```python
from build123d import *

# Parameters (mm, degrees)
F1_DEPTH = 2
F2_R     = 1
F3_DEPTH = 2.001


with BuildPart() as f1:
    # F0 (on Top) → F1 (new body)
    with BuildSketch(Plane.XY):
        with BuildLine():
            ThreePointArc((9.772306, -2.121802), (9.942913, -1.066992), (10, 0))
            ThreePointArc((10, 0), (9.999976, 0.02183), (9.999905, 0.043659))
            ThreePointArc((9.999905, 0.043659), (9.945219, 1.045285), (9.79046, 2.036392))
            ThreePointArc((9.79046, 2.036392), (9.510565, 3.09017), (9.11761, 4.107212))
            ThreePointArc((9.11761, 4.107212), (8.660254, 5), (8.115755, 5.842476))
            ThreePointArc((8.115755, 5.842476), (7.431448, 6.691306), (6.658797, 7.460591))
            ThreePointArc((6.658797, 7.460591), (5.877853, 8.09017), (5.037762, 8.638342))
            ThreePointArc((5.037762, 8.638342), (4.067366, 9.135455), (3.048618, 9.523966))
            ThreePointArc((3.048618, 9.523966), (2.079117, 9.781476), (1.088694, 9.940561))
            ThreePointArc((1.088694, 9.940561), (0, 10), (-1.088694, 9.940561))
            ThreePointArc((-1.088694, 9.940561), (-2.079117, 9.781476), (-3.048618, 9.523966))
            ThreePointArc((-3.048618, 9.523966), (-4.067366, 9.135455), (-5.037762, 8.638342))
            ThreePointArc((-5.037762, 8.638342), (-5.877853, 8.09017), (-6.658797, 7.460591))
            ThreePointArc((-6.658797, 7.460591), (-7.431448, 6.691306), (-8.115755, 5.842476))
            ThreePointArc((-8.115755, 5.842476), (-8.660254, 5), (-9.11761, 4.107212))
            ThreePointArc((-9.11761, 4.107212), (-9.510565, 3.09017), (-9.79046, 2.036392))
            ThreePointArc((-9.79046, 2.036392), (-9.945219, 1.045285), (-9.999905, 0.043659))
            ThreePointArc((-9.999905, 0.043659), (-9.945219, -1.045285), (-9.772306, -2.121802))
            ThreePointArc((-9.772306, -2.121802), (-9.510565, -3.09017), (-9.153125, -4.027443))
            ThreePointArc((-9.153125, -4.027443), (-8.660254, -5), (-8.064431, -5.913117))
            ThreePointArc((-8.064431, -5.913117), (-7.431448, -6.691306), (-6.723687, -7.402164))
            ThreePointArc((-6.723687, -7.402164), (-5.877853, -8.09017), (-4.962143, -8.682001))
            ThreePointArc((-4.962143, -8.682001), (-4.067366, -9.135455), (-3.131663, -9.496983))
            ThreePointArc((-3.131663, -9.496983), (-2.079117, -9.781476), (-1.001855, -9.949688))
            ThreePointArc((-1.001855, -9.949688), (0, -10), (1.001855, -9.949688))
            ThreePointArc((1.001855, -9.949688), (2.079117, -9.781476), (3.131663, -9.496983))
            ThreePointArc((3.131663, -9.496983), (4.067366, -9.135455), (4.962143, -8.682001))
            ThreePointArc((4.962143, -8.682001), (5.877853, -8.09017), (6.723687, -7.402164))
            ThreePointArc((6.723687, -7.402164), (7.431448, -6.691306), (8.064431, -5.913117))
            ThreePointArc((8.064431, -5.913117), (8.660254, -5), (9.153125, -4.027443))
            ThreePointArc((9.153125, -4.027443), (9.510565, -3.09017), (9.772306, -2.121802))
        make_face()
        with BuildLine():
            ThreePointArc((9.999905, 0.043659), (9.999976, 0.02183), (10, 0))
            ThreePointArc((10, 0), (9.942913, -1.066992), (9.772306, -2.121802))
            ThreePointArc((9.772306, -2.121802), (10.85461, -2.093182), (11.881999, -1.751603))
            Line((11.881999, -1.751603), (11.934263, -1.254342))
            Line((11.934263, -1.254342), (11.986527, -0.757081))
            ThreePointArc((11.986527, -0.757081), (11.052608, -0.209359), (9.999905, 0.043659))
        make_face()
        with BuildLine():
            ThreePointArc((9.11761, 4.107212), (9.510565, 3.09017), (9.79046, 2.036392))
            ThreePointArc((9.79046, 2.036392), (10.767554, 2.502751), (11.567187, 3.232676))
            Line((11.567187, 3.232676), (11.412678, 3.708204))
            Line((11.412678, 3.708204), (11.25817, 4.183732))
            ThreePointArc((11.25817, 4.183732), (10.182214, 4.304241), (9.11761, 4.107212))
        make_face()
        with BuildLine():
            ThreePointArc((10.642305, -5.566987), (10.011906, -4.68676), (9.153125, -4.027443))
            ThreePointArc((9.153125, -4.027443), (8.660254, -5), (8.064431, -5.913117))
            ThreePointArc((8.064431, -5.913117), (9.064806, -6.327185), (10.142305, -6.433013))
            Line((10.142305, -6.433013), (10.392305, -6))
            Line((10.392305, -6), (10.642305, -5.566987))
        make_face()
        with BuildLine():
            ThreePointArc((6.658797, 7.460591), (7.431448, 6.691306), (8.115755, 5.842476))
            ThreePointArc((8.115755, 5.842476), (8.818689, 6.665935), (9.252303, 7.657995))
            Line((9.252303, 7.657995), (8.917738, 8.029567))
            Line((8.917738, 8.029567), (8.583173, 8.40114))
            ThreePointArc((8.583173, 8.40114), (7.551223, 8.0736), (6.658797, 7.460591))
        make_face()
        with BuildLine():
            ThreePointArc((7.457932, -9.414311), (7.240054, -8.353777), (6.723687, -7.402164))
            ThreePointArc((6.723687, -7.402164), (5.877853, -8.09017), (4.962143, -8.682001))
            ThreePointArc((4.962143, -8.682001), (5.707615, -9.46716), (6.648915, -10.002097))
            Line((6.648915, -10.002097), (7.053423, -9.708204))
            Line((7.053423, -9.708204), (7.457932, -9.414311))
        make_face()
        with BuildLine():
            ThreePointArc((3.048618, 9.523966), (4.067366, 9.135455), (5.037762, 8.638342))
            ThreePointArc((5.037762, 8.638342), (5.344994, 9.676519), (5.337612, 10.759177))
            Line((5.337612, 10.759177), (4.88084, 10.962545))
            Line((4.88084, 10.962545), (4.424067, 11.165914))
            ThreePointArc((4.424067, 11.165914), (3.614556, 10.446959), (3.048618, 9.523966))
        make_face()
        with BuildLine():
            ThreePointArc((2.984014, -11.633815), (3.216331, -10.576351), (3.131663, -9.496983))
            ThreePointArc((3.131663, -9.496983), (2.079117, -9.781476), (1.001855, -9.949688))
            ThreePointArc((1.001855, -9.949688), (1.363525, -10.970177), (2.005866, -11.841727))
            Line((2.005866, -11.841727), (2.49494, -11.737771))
            Line((2.49494, -11.737771), (2.984014, -11.633815))
        make_face()
        with BuildLine():
            ThreePointArc((-1.088694, 9.940561), (0, 10), (1.088694, 9.940561))
            ThreePointArc((1.088694, 9.940561), (0.9471, 11.013945), (0.5, 12))
            Line((0.5, 12), (0, 12))
            Line((0, 12), (-0.5, 12))
            ThreePointArc((-0.5, 12), (-0.9471, 11.013945), (-1.088694, 9.940561))
        make_face()
        with BuildLine():
            ThreePointArc((-2.005866, -11.841727), (-1.363525, -10.970177), (-1.001855, -9.949688))
            ThreePointArc((-1.001855, -9.949688), (-2.079117, -9.781476), (-3.131663, -9.496983))
            ThreePointArc((-3.131663, -9.496983), (-3.216331, -10.576351), (-2.984014, -11.633815))
            Line((-2.984014, -11.633815), (-2.49494, -11.737771))
            Line((-2.49494, -11.737771), (-2.005866, -11.841727))
        make_face()
        with BuildLine():
            ThreePointArc((-5.037762, 8.638342), (-4.067366, 9.135455), (-3.048618, 9.523966))
            ThreePointArc((-3.048618, 9.523966), (-3.614556, 10.446959), (-4.424067, 11.165914))
            Line((-4.424067, 11.165914), (-4.88084, 10.962545))
            Line((-4.88084, 10.962545), (-5.337612, 10.759177))
            ThreePointArc((-5.337612, 10.759177), (-5.344994, 9.676519), (-5.037762, 8.638342))
        make_face()
        with BuildLine():
            ThreePointArc((-6.648915, -10.002097), (-5.707615, -9.46716), (-4.962143, -8.682001))
            ThreePointArc((-4.962143, -8.682001), (-5.877853, -8.09017), (-6.723687, -7.402164))
            ThreePointArc((-6.723687, -7.402164), (-7.240054, -8.353777), (-7.457932, -9.414311))
            Line((-7.457932, -9.414311), (-7.053423, -9.708204))
            Line((-7.053423, -9.708204), (-6.648915, -10.002097))
        make_face()
        with BuildLine():
            ThreePointArc((-8.115755, 5.842476), (-7.431448, 6.691306), (-6.658797, 7.460591))
            ThreePointArc((-6.658797, 7.460591), (-7.551223, 8.0736), (-8.583173, 8.40114))
            Line((-8.583173, 8.40114), (-8.917738, 8.029567))
            Line((-8.917738, 8.029567), (-9.252303, 7.657995))
            ThreePointArc((-9.252303, 7.657995), (-8.818689, 6.665935), (-8.115755, 5.842476))
        make_face()
        with BuildLine():
            ThreePointArc((-10.142305, -6.433013), (-9.064806, -6.327185), (-8.064431, -5.913117))
            ThreePointArc((-8.064431, -5.913117), (-8.660254, -5), (-9.153125, -4.027443))
            ThreePointArc((-9.153125, -4.027443), (-10.011906, -4.68676), (-10.642305, -5.566987))
            Line((-10.642305, -5.566987), (-10.392305, -6))
            Line((-10.392305, -6), (-10.142305, -6.433013))
        make_face()
        with BuildLine():
            ThreePointArc((-9.79046, 2.036392), (-9.510565, 3.09017), (-9.11761, 4.107212))
            ThreePointArc((-9.11761, 4.107212), (-10.182214, 4.304241), (-11.25817, 4.183732))
            Line((-11.25817, 4.183732), (-11.412678, 3.708204))
            Line((-11.412678, 3.708204), (-11.567187, 3.232676))
            ThreePointArc((-11.567187, 3.232676), (-10.767554, 2.502751), (-9.79046, 2.036392))
        make_face()
        with BuildLine():
            ThreePointArc((-11.881999, -1.751603), (-10.85461, -2.093182), (-9.772306, -2.121802))
            ThreePointArc((-9.772306, -2.121802), (-9.945219, -1.045285), (-9.999905, 0.043659))
            ThreePointArc((-9.999905, 0.043659), (-11.052608, -0.209359), (-11.986527, -0.757081))
            Line((-11.986527, -0.757081), (-11.934263, -1.254342))
            Line((-11.934263, -1.254342), (-11.881999, -1.751603))
        make_face()
    extrude(amount=F1_DEPTH)

    # F2 (on face) → F3 (cut, through all)
    with BuildSketch(Plane.XY.offset(2)):
        Circle(F2_R)
    extrude(amount=-F3_DEPTH, mode=Mode.SUBTRACT)


solid = f1.part
```
Design review of the part built by this model. Coordinates are the model's own, in mm. A direction names the side the tool comes from. Coordinates: 2 decimals unless noted, no trailing zeros. Order: outer loops, then holes, each group sorted by start corner. A loop starts at its lowest first (then second) coordinate and runs counter-clockwise, first axis right, second up. Notation, with made-up numbers: (26, 86) - (58, 86) arc R18 ccw to (58, 99) - close; hole circle Ø2 at (58, 53). An arc over 180 degrees is marked (long way). One line per question, with ' | ' between items.
Q1. Consider section B-B, the plane y = -10.5. Give the boundary of the cut face in (x, z), then the cut area to 3 significant figures.
Answer key:
outline: (-3.22, 0) - (-1.15, 0) - (-1.15, 2) - (-3.22, 2) - close; (1.15, 0) - (3.22, 0) - (3.22, 2) - (1.15, 2) - close | area: 8.26 mm2
Q2. Consider section A-A, the plane x = 0. Give the boundary of the cut face in (y, z).
Answer key:
outline: (-10, 0) - (-1, 0) - (-1, 2) - (-10, 2) - close; (1, 0) - (12, 0) - (12, 2) - (1, 2) - close
Q3. Clearance check with a flat-ended pin moving along its axis: pin 1 Ø6 at (x, y) = (3.5, -3.5) entering from -Z. State where the tip first meets the part, or that it passes through.
Answer key:
pin 1: stops at z = 0
Q4. The part is to be moulded in two halves that separate along X. For faces 1 (the cylindrical face through (-7.235, -8.339, 0.986)), 2 (the flat face through (0, 12, 1)), 3 (the cylindrical face through (3.215, -10.592, 0.986)), say which applies: +X half, -X half, draft (parallel to the pull), parting line (faces both ways), or undercut.
Answer key:
face 1: -X half | face 2: draft | face 3: undercut
Q5. Consider section D-D, the plane y = -5. Give the boundary of the cut face in (x, z), then the cut area to 3 significant figures.
Answer key:
outline: (-10.28, 0) - (10.28, 0) - (10.28, 2) - (-10.28, 2) - close | area: 41.1 mm2
Q6. To check wall thickness, follow line 1 along X through (y, z) = (10.5, 1); line 2 along Y through (x, z) = (0, 0.7); line 3 along X through (y, z) = (-9, 1.05). State the ranges of each line that lie inside material, in increasing order.
Answer key:
line 1: x = -5.37 to -3.66, -1.06 to 1.06, 3.66 to 5.37 | line 2: y = -10 to -1, 1 to 12 | line 3: x = -7.41 to -5.21, -4.36 to 4.36, 5.21 to 7.41
Q7. For faces 4 (the cylindrical face through (-10.001, -4.676, 0.986)), 5 (the cylindrical face through (9.947, 1.031, 0.986)), 6 (the cylindrical face through (3.624, 10.459, 0.986)), 7 (the cylindrical face through (7.422, -6.702, 0.986)), 8 (the cylindrical face through (-5.72, -9.477, 0.986)), list the 3-axis set-ups (+Z, -Z, +X, -X, +Y, -Y) from which the entire face can be reached by the end or side of a thin tool; tool diameter is ignored.
Answer key:
face 4: +Z, -Z, -X | face 5: +Z, -Z, +X | face 6: +Z, -Z, +Y | face 7: +Z, -Z | face 8: +Z, -Z, -Y
Q8. Consider section C-C, the plane x = -7.75. Give the boundary of the cut face in (y, z).
Answer key:
outline: (-6.32, 0) - (8.16, 0) - (8.16, 2) - (-6.32, 2) - close
